The model under review builds one solid part; all positions refer to its coordinate system, in mm. A direction names the side the tool comes from. Coordinates: 2 decimals unless noted, no trailing zeros. Order: outer loops, then holes, each group sorted by start corner. A loop starts at its lowest first (then second) coordinate and runs counter-clockwise, first axis right, second up. Notation, with made-up numbers: M 70,22.25 L 74,22.25 A26 cw 74,51.25 Z; hole C 7.25,9.5 d7. An arc over 180 degrees is marked long. Answer as CSV lines item,"result". Start each with the question number.
Q1. Consider section D-D on x = 20. Write out the cut boundary in (y, z), and give its area (3 significant figures).
Q2. Consider section A-A on x = -13.5. Write out the cut boundary in (y, z), and give its area (3 significant figures).
Q3. Wall thickness on L1, parallel to Y at x = 23.5, z = 1.45; L2, parallel to Y at x = 5.5, z = 3.55; L3, parallel to Y at x = 20.5, z = 3.9: over which ranges is each line inside the solid? List them lowest first. Write a range as [from, to].
Q4. Consider section B-B on x = -23.5. Write out the cut boundary in (y, z).
Q5. The part is to be moulded in two halves that separate along X. For faces 1 (the face through (1.6, 7.93, 2.46)), 2 (the face through (0, 3, 5)), 3 (the face through (-26.93, -11.9, 2.54)), 4 (the face through (26.9, -11.93, 2.54)), say which applies: +X half, -X half, draft (parallel to the pull), parting line (faces both ways), or undercut.
Q6. Machinability: for faces 5 (the face through (26.9, 11.93, 2.54)), 6 (the face through (-1.298, 4.716, 2.465)), which of the approach directions +Z, -Z, +X, -X, +Y, -Y give a long, thin tool a straight path to every point of the face, cutting with its end or side? Answer none if there is none.
Q7. For P1, Ø8, axis at x = -15, y = -8, coming from the -Z side, flat-tipped, find the tip position at first contact; note if it passes through.
Q8. Consider section C-C on y = -4.5. Write out the cut boundary in (x, z), and give its area (3 significant figures).
from build123d import *

# Parameters (mm, degrees)
SKETCH_1_W          = 55
SKETCH_1_H          = 25
EXTRUDE_1_DEPTH     = 5
SKETCH_2_R          = 1.5
CUT_EXTRUDE_1_DEPTH = 5
CUT_EXTRUDE_2_DEPTH = 5
FILLET_1_R          = 2
FILLET_2_R          = 2


with BuildPart() as part:
    # 草图1 → 凸台-拉伸1 (new body)
    with BuildSketch(Plane.XY):
        Rectangle(SKETCH_1_W, SKETCH_1_H)
    extrude(amount=EXTRUDE_1_DEPTH)

    # 草图2 → 切除-拉伸1 (cut)
    with BuildSketch(Plane.XY.offset(5)):
        with Locations((-23.5, 0)):
            Circle(SKETCH_2_R)
        Circle(SKETCH_2_R)
        with Locations((23.5, 0)):
            Circle(SKETCH_2_R)
    extrude(amount=-CUT_EXTRUDE_1_DEPTH, mode=Mode.SUBTRACT)

    # 草图3 → 切除-拉伸2 (cut)
    with BuildSketch(Plane.XY.offset(5)):
        with BuildLine():
            Line((-22.5, -4.387482194), (-22.5, -8.5))
            Line((-22.5, -8.5), (-1, -8.5))
            Line((-1, -8.5), (-1, -4.387482194))
            ThreePointArc((-1, -4.387482194), (-4.5, 0), (-1, 4.387482194))
            Line((-1, 4.387482194), (-1, 8.5))
            Line((-1, 8.5), (-22.5, 8.5))
            Line((-22.5, 8.5), (-22.5, 4.387482194))
            ThreePointArc((-22.5, 4.387482194), (-19.98218818, 2.80624304), (-19, 0))
            ThreePointArc((-19, 0), (-19.98218818, -2.80624304), (-22.5, -4.387482194))
        make_face()
    cut_extrude_2 = extrude(amount=-CUT_EXTRUDE_2_DEPTH, mode=Mode.SUBTRACT)

    # 镜向2: 切除-拉伸2 across plane
    add(cut_extrude_2.mirror(Plane(origin=(0, 0, 0), x_dir=(0, 0, 1), z_dir=(1, 0, 0))), mode=Mode.SUBTRACT)

    # 圆角1
    fillet_1_edges = [part.edges().sort_by_distance(p)[0] for p in [
        (-1, 4.387482194, 2.5),
        (-1, -4.387482194, 2.5),
        (-1, -8.5, 2.5),
        (-22.5, -8.5, 2.5),
        (-22.5, -4.387482194, 2.5),
        (-22.5, 4.387482194, 2.5),
        (-22.5, 8.5, 2.5),
        (-1, 8.5, 2.5),
        (1, -4.387482194, 2.5),
        (1, 4.387482194, 2.5),
        (1, 8.5, 2.5),
        (22.5, 8.5, 2.5),
        (22.5, 4.387482194, 2.5),
        (22.5, -4.387482194, 2.5),
        (22.5, -8.5, 2.5),
        (1, -8.5, 2.5),
    ]]
    fillet(fillet_1_edges, radius=FILLET_1_R)

    # 圆角2
    fillet_2_edges = [part.edges().sort_by_distance(p)[0] for p in [
        (27.5, -12.5, 2.5),
        (-27.5, -12.5, 2.5),
        (-27.5, 12.5, 2.5),
        (27.5, 12.5, 2.5),
    ]]
    fillet(fillet_2_edges, radius=FILLET_2_R)


solid = part.part
Evaluation:
1,outline,"M -12.5,0 L -8.5,0 L -8.5,5 L -12.5,5 Z; M -2.83,0 L 2.83,0 L 2.83,5 L -2.83,5 Z; M 8.5,0 L 12.5,0 L 12.5,5 L 8.5,5 Z"
1,area,"68.3 mm²"
2,outline,"M -12.5,0 L -8.5,0 L -8.5,5 L -12.5,5 Z; M 8.5,0 L 12.5,0 L 12.5,5 L 8.5,5 Z"
2,area,"40.0 mm²"
3,L1,"y = [-12.5, -1.5], [1.5, 12.5]"
3,L2,"y = [-12.5, -8.5], [8.5, 12.5]"
3,L3,"y = [-12.5, -8.5], [-3.35, 3.35], [8.5, 12.5]"
4,outline,"M -12.5,0 L -1.5,0 L -1.5,5 L -12.5,5 Z; M 1.5,0 L 12.5,0 L 12.5,5 L 1.5,5 Z"
5,face 1,"undercut"
5,face 2,"draft"
5,face 3,"-X half"
5,face 4,"+X half"
6,face 5,"+Z, -Z, +X, +Y"
6,face 6,"+Z, -Z"
7,P1,"stops at z = 0"
8,outline,"M -27.5,0 L -22.05,0 L -22.05,5 L -27.5,5 Z; M -1.45,0 L 1.45,0 L 1.45,5 L -1.45,5 Z; M 22.05,0 L 27.5,0 L 27.5,5 L 22.05,5 Z"
8,area,"69.0 mm²"
